Work out the finished part from the listing and answer in its coordinate system (mm). A direction names the side the tool comes from. Coordinates: 2 decimals unless noted, no trailing zeros. Loops run counter-clockwise (first coordinate to the right, second up) from the corner with the lowest first, then second, coordinate; pieces in that order, holes last. Notation, with made-up numbers: (37.25, 64) -> (87.25, 64) arc R19 cw to (87.25, 98) -> close; hole circle Ø10 at (-29.5, 0). An arc over 180 degrees is marked (long way). Use a Markdown table: item, result. Add a question column.
```python
from build123d import *

# Parameters (mm, degrees)
F0_W     = 80
F0_H     = 80
F0_R     = 2
F0_R_2   = 35.75
F1_DEPTH = 25
F2_R     = 6
F5_DEPTH = 11


with BuildPart() as f1:
    # F0 (on Top) → F1 (new body)
    with BuildSketch(Plane.XY):
        Rectangle(F0_W, F0_H)
        with Locations((-35.75, -35.75)):
            Circle(F0_R, mode=Mode.SUBTRACT)
        with Locations((35.75, -35.75)):
            Circle(F0_R, mode=Mode.SUBTRACT)
        with Locations((-35.75, 35.75)):
            Circle(F0_R, mode=Mode.SUBTRACT)
        Circle(F0_R_2, mode=Mode.SUBTRACT)
        with Locations((35.75, 35.75)):
            Circle(F0_R, mode=Mode.SUBTRACT)
    extrude(amount=F1_DEPTH)

    # F2
    f2_edges = [f1.edges().sort_by_distance(p)[0] for p in [
        (-40, -40, 12.5),
        (40, -40, 12.5),
        (40, 40, 12.5),
        (-40, 40, 12.5),
    ]]
    fillet(f2_edges, radius=F2_R)

    # F4 (on offset) → F5 (cut)
    with BuildSketch(Plane.XY.offset(7)):
        with BuildLine():
            ThreePointArc((0, 42), (29.6984848098, 29.6984848098), (42, 0))
            Line((42, 0), (42, 42))
            Line((42, 42), (0, 42))
        make_face()
        with BuildLine():
            ThreePointArc((-42, 5.59e-08), (-29.6984847901, 29.6984848296), (0, 42))
            Line((0, 42), (-42, 42))
            Line((-42, 42), (-42, 5.59e-08))
        make_face()
        with BuildLine():
            Line((-42, -42), (1.331e-07, -42))
            ThreePointArc((1.331e-07, -42), (-29.6984847825, -29.6984848372), (-42, 5.59e-08))
            Line((-42, 5.59e-08), (-42, -42))
        make_face()
        with BuildLine():
            Line((42, -42), (42, 0))
            ThreePointArc((42, 0), (29.6984848569, -29.6984847628), (1.331e-07, -42))
            Line((1.331e-07, -42), (42, -42))
        make_face()
    extrude(amount=F5_DEPTH, mode=Mode.SUBTRACT)


solid = f1.part
```
Item 1: Section D-D (x = 21) is taken. Determine the outline of the cut face in (y, z), then the cut area to 3 significant figures.
Item 2: For a pull along Z with two mould halves and no side action, classify faces 1 (the face through (29.5, 29.896, 12.423)), 2 (the face through (36.673, -37.524, 3.451)) as +Z half, -Z half, draft (parallel to the pull), parting line (faces both ways), or undercut.
Item 3: Find the intervals of material crossed by probe 1 along Z at (x, y) = (-34, 34.5); probe 2 along X at (y, z) = (-36, 2.25); probe 3 along Y at (x, z) = (6, 8.5), in increasing order.
Item 4: Section C-C (z = 17) is taken. Determine the outline of the cut face in (x, y), then the cut area to 3 significant figures.
Item 5: For faces 3 (the face through (29.896, -29.5, 12.423)), 4 (the face through (-29.896, 29.5, 12.423)), 5 (the face through (32, 34, 7)), determine the directions among +Z, -Z, +X, -X, +Y, -Y from which every point of the face is accessible in a straight line to the end or side of a thin tool.
Item 6: Section A-A (y = 0) is taken. Determine the outline of the cut face in (x, z).
Item 7: Given pin 1 (22 mm diameter, centred on x = 22.5, y = -26.5, fed in from +Z); pin 2 (1.5 mm diameter, centred on y = 24.5, z = 13.5, fed in from -X), each flat-ended and moving along its own axis, determine where each tip first touches the part or whether it passes through.
Output:
| question | item | result |
|---|---|---|
| 1 | outline | (-40, 0) -> (-28.93, 0) -> (-28.93, 25) -> (-40, 25) -> (-40, 18) -> (-36.37, 18) -> (-36.37, 7) -> (-40, 7) -> close; (28.93, 0) -> (40, 0) -> (40, 7) -> (36.37, 7) -> (36.37, 18) -> (40, 18) -> (40, 25) -> (28.93, 25) -> close |
| 1 | area | 474 mm2 |
| 2 | face 1 | undercut |
| 2 | face 2 | draft |
| 3 | probe 1 | z = 0 to 7, 18 to 25 |
| 3 | probe 2 | x = -39.66 to -37.73, -33.77 to 33.77, 37.73 to 39.66 |
| 3 | probe 3 | y = -40 to -35.24, 35.24 to 40 |
| 4 | outline | (-40, -12.81) arc R42 ccw to (-12.81, -40) -> (12.81, -40) arc R42 ccw to (40, -12.81) -> (40, 12.81) arc R42 ccw to (12.81, 40) -> (-12.81, 40) arc R42 ccw to (-40, 12.81) -> close; hole circle Ø71.5 at (0, 0) |
| 4 | area | 1,390 mm2 |
| 5 | face 3 | +X, -Y |
| 5 | face 4 | -X, +Y |
| 5 | face 5 | +X, +Y |
| 6 | outline | (-40, 0) -> (-35.75, 0) -> (-35.75, 25) -> (-40, 25) -> close; (35.75, 0) -> (40, 0) -> (40, 25) -> (35.75, 25) -> close |
| 7 | pin 1 | stops at z = 25 |
| 7 | pin 2 | stops at x = -34.64 |
